Work out the finished part from the listing and answer in its coordinate system (mm). A direction names the side the tool comes from. Give positions to 0.01 mm unless a question says otherwise; leave off trailing zeros. Loops run counter-clockwise (first coordinate to the right, second up) from the corner with the lowest first, then second, coordinate; pieces in that order, holes last. Notation, with made-up numbers: (-5.5, 61.5) - (20.5, 61.5) arc R21 ccw to (20.5, 92.5) - close; hole circle Ø2 at (6.5, 53.25). An arc over 180 degrees is marked (long way). Use one line per item in the form item = value. Start each with the question number.
from build123d import *

# Parameters (mm, degrees)
SKETCH_1_W         = 32
SKETCH_1_H         = 32
SKETCH_1_R         = 1.25
EXTRUDE_1463_DEPTH = 1.5
EXTRUDE_START      = 1.5
SKETCH_1_3_W       = 22.3
SKETCH_1_3_H       = 5.5
EXTRUDE_1638_DEPTH = 2.5
SKETCH_1_4_R       = 6.9
SKETCH_1_4_R_2     = 6
EXTRUDE_1808_DEPTH = 8
EXTRUDE_START_2    = 9.5
SKETCH_1_5_R       = 6
EXTRUDE_1980_DEPTH = 3.5
EXTRUDE_START_3    = 13
SKETCH_1_6_R       = 7.75
SKETCH_1_6_R_2     = 6.9
SKETCH_1_6_R_3     = 6
EXTRUDE_2074_DEPTH = 5.5
SKETCH_1_7_R       = 1.5
EXTRUDE_2255_DEPTH = 0.5
SKETCH_2_W         = 16
SKETCH_2_H         = 1
EXTRUDE_2715_DEPTH = 10
SKETCH_3_W         = 16
SKETCH_3_H         = 1
EXTRUDE_3012_DEPTH = 10


with BuildPart() as part:
    # Эскиз1 → Extrude 1463 (new body)
    with BuildSketch(Plane.XY):
        Rectangle(SKETCH_1_W, SKETCH_1_H)
        with Locations((-14.25, -14.25)):
            Circle(SKETCH_1_R, mode=Mode.SUBTRACT)
        with Locations((14.25, -14.25)):
            Circle(SKETCH_1_R, mode=Mode.SUBTRACT)
        with Locations((-14.25, 14.25)):
            Circle(SKETCH_1_R, mode=Mode.SUBTRACT)
        with Locations((14.25, 14.25)):
            Circle(SKETCH_1_R, mode=Mode.SUBTRACT)
    extrude(amount=EXTRUDE_1463_DEPTH)

    # Эскиз1<3> → Extrude 1638 (add)
    with BuildSketch(Plane.XY.offset(EXTRUDE_START)):
        with Locations((0, -13.25)):
            Rectangle(SKETCH_1_3_W, SKETCH_1_3_H)
    extrude(amount=EXTRUDE_1638_DEPTH)

    # Эскиз1<4> → Extrude 1808 (add)
    # profile 1 of 2: a face of its own
    with BuildSketch(Plane.XY.offset(EXTRUDE_START)):
        Circle(SKETCH_1_4_R)
        Circle(SKETCH_1_4_R_2, mode=Mode.SUBTRACT)
    # profile 2 of 2: a face of its own
    with BuildSketch(Plane.XY.offset(EXTRUDE_START)):
        Circle(SKETCH_1_4_R_2)
    extrude(amount=EXTRUDE_1808_DEPTH)

    # Эскиз1<5> → Extrude 1980 (add)
    with BuildSketch(Plane.XY.offset(EXTRUDE_START_2)):
        Circle(SKETCH_1_5_R)
    extrude(amount=EXTRUDE_1980_DEPTH)

    # Эскиз1<6> → Extrude 2074 (add)
    # profile 1 of 3: a face of its own
    with BuildSketch(Plane.XY.offset(EXTRUDE_START_3)):
        Circle(SKETCH_1_6_R)
        Circle(SKETCH_1_6_R_2, mode=Mode.SUBTRACT)
    # profile 2 of 3: a face of its own
    with BuildSketch(Plane.XY.offset(EXTRUDE_START_3)):
        Circle(SKETCH_1_6_R_2)
        Circle(SKETCH_1_6_R_3, mode=Mode.SUBTRACT)
    # profile 3 of 3: a face of its own
    with BuildSketch(Plane.XY.offset(EXTRUDE_START_3)):
        Circle(SKETCH_1_6_R_3)
    extrude(amount=EXTRUDE_2074_DEPTH)

    # Эскиз1<7> → Extrude 2255 (add)
    with BuildSketch(Plane.XY):
        with Locations((9.5, 0)):
            Circle(SKETCH_1_7_R)
        with Locations((-9.5, 0)):
            Circle(SKETCH_1_7_R)
    extrude(amount=-EXTRUDE_2255_DEPTH)

    # Эскиз2 → Extrude 2715 (add)
    with BuildSketch(Plane.XZ.offset(16)):
        with Locations((0, 3)):
            Rectangle(SKETCH_2_W, SKETCH_2_H)
    extrude(amount=EXTRUDE_2715_DEPTH)

    # Эскиз3 → Extrude 3012 (add)
    with BuildSketch(Plane(origin=(0, 0, 2.5), x_dir=(-1, 0, 0), z_dir=(0, 0, -1))):
        with Locations((0, -25.5)):
            Rectangle(SKETCH_3_W, SKETCH_3_H)
    extrude(amount=EXTRUDE_3012_DEPTH)


solid = part.part
1) Determine the mould class of faces 1 (the flat face through (0.1, -25.5, -7.5)), 2 (the cylindrical face through (-0.9, 6.84, 5.44)), 3 (the flat face through (0, -16, 2)) for opening direction Z: released by +Z, released by -Z, zero draft, split by the parting line, or undercut.
2) A tool of negligible diameter and unlimited length cuts with its end or side. For faces 4 (the cylindrical face through (8, 0.07, -0.25)), 5 (the flat face through (4, -5, 13)), 6 (the flat face through (0, -25, -2)), 7 (the flat face through (-8, -23, 3)), 8 (the flat face through (0, -13, 4)), from which of +Z, -Z, +X, -X, +Y, -Y can it reach the whole face along a straight path? Write none if from no direction.
3) A cutting plane is placed at D-D (y = -14.25). Give the vertices of the cut face in (x, z), plus the area to 4 significant figures.
4) Find the intervals of material crossed by probe 1 along Y at (x, z) = (14.25, 0.6); probe 2 along Z at (x, y) = (6, -2); probe 3 along Z at (x, y) = (3, 11), in increasing order.
5) A cutting plane is placed at A-A (y = 14.25). Give the vertices of the cut face in (x, z).
6) Flat-ended cylindrical pins translate along their axes: pin 1 Ø4.5 at (x, y) = (0, -0.5) entering from -Z; pin 2 Ø5 at (y, z) = (-21, -1) entering from -X; pin 3 Ø1 at (x, y) = (8, -17.5) entering from -Z; pin 4 Ø2.5 at (x, y) = (-10, 0) entering from -Z. Find the tip coordinate at first contact, or state that the pin passes through.
7) A cutting plane is placed at B-B (x = 0). Give the vertices of the cut face in (y, z), plus the area to 3 significant figures.
Answer sheet:
q1.face_1 = released by -Z
q1.face_2 = undercut
q1.face_3 = zero draft
q2.face_4 = -Z
q2.face_5 = none
q2.face_6 = -Z, +X, -X
q2.face_7 = +Z, -Z, -X, -Y
q2.face_8 = +Z, +X, -X, -Y
q3.outline = (-16, 0) - (-15.5, 0) - (-15.5, 1.5) - (-16, 1.5) - close; (-13, 0) - (13, 0) - (13, 1.5) - (11.15, 1.5) - (11.15, 4) - (-11.15, 4) - (-11.15, 1.5) - (-13, 1.5) - close; (15.5, 0) - (16, 0) - (16, 1.5) - (15.5, 1.5) - close
q3.area = 96.25 mm²
q4.probe_1 = -16 to -15.5, -13 to 13, 15.5 to 16
q4.probe_2 = 0 to 9.5, 13 to 18.5
q4.probe_3 = 0 to 1.5
q5.outline = (-16, 0) - (-15.5, 0) - (-15.5, 1.5) - (-16, 1.5) - close; (-13, 0) - (13, 0) - (13, 1.5) - (-13, 1.5) - close; (15.5, 0) - (16, 0) - (16, 1.5) - (15.5, 1.5) - close
q6.pin_1 = 0
q6.pin_2 = through
q6.pin_3 = 2.5
q6.pin_4 = -0.5
q7.outline = (-26, -7.5) - (-25, -7.5) - (-25, 2.5) - (-16, 2.5) - (-16, 0) - (16, 0) - (16, 1.5) - (6.9, 1.5) - (6.9, 9.5) - (6, 9.5) - (6, 13) - (7.75, 13) - (7.75, 18.5) - (-7.75, 18.5) - (-7.75, 13) - (-6, 13) - (-6, 9.5) - (-6.9, 9.5) - (-6.9, 1.5) - (-10.5, 1.5) - (-10.5, 4) - (-16, 4) - (-16, 3.5) - (-26, 3.5) - close
q7.area = 319 mm²
